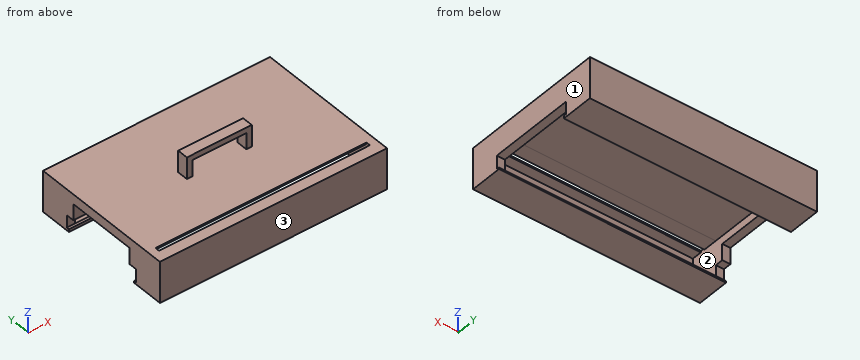
Solid Edge part; units mm, degrees
sketch "Sketch1" plane through (0, 0, 0) normal (0, 0, 1) x (1, 0, 0)
  line L0 (-210, -135) -> (210, -135)
  line L1 (210, -135) -> (210, 135)
  line L2 (210, 135) -> (-210, 135)
  line L3 (-210, 135) -> (-210, -135)
extrude "Protrusion1" add sketch "Sketch1" along normal blind 76
sketch "Sketch2" plane through (0, 0, 0) normal (0, 0, -1) x (1, 0, 0)
  line L0 (-195, 80) -> (195, 80)
  line L1 (195, 80) -> (195, -80)
  line L2 (195, -80) -> (-195, -80)
  line L3 (-195, -80) -> (-195, 80)
extrude "ExtrudedCutout_1" cut sketch "Sketch2" against normal blind 70
sketch "Sketch3" plane through (0, -80, 35) normal (0, 1, 0) x (-1, 0, 0)
  line L0 (195, -32) -> (-195, -32)
  line L1 (-195, -32) -> (-195, 38)
  line L2 (-195, 38) -> (195, 38)
  line L3 (195, 38) -> (195, -32)
extrude "ExtrudedCutout_2" cut sketch "Sketch3" against normal blind 53
sketch "Sketch4" plane through (210, 0, 38) normal (1, 0, 0) x (0, 1, 0)
  line L0 (80, -10) -> (-80, -10)
  line L1 (-80, -10) -> (-80, -38)
  line L2 (-80, -38) -> (80, -38)
  line L3 (80, -38) -> (80, -10)
extrude "Cutout1" cut sketch "Sketch4" against normal through all
sketch "Sketch5" plane through (0, 0, 70) normal (0, 0, -1) x (0, 1, 0)
  line L0 (80, -195) -> (-80, -195)
  line L1 (-80, -195) -> (-80, 195)
  line L2 (-80, 195) -> (80, 195)
  line L3 (80, 195) -> (80, -195)
extrude "ExtrudedCutout_5" cut sketch "Sketch5" against normal blind 2.5929
sketch "Sketch6" plane through (0, 0, 70) normal (0, 0, -1) x (0, 1, 0)
  line L0 (80, -195) -> (-80, -195)
  line L1 (-80, -195) -> (-80, 195)
  line L2 (-80, 195) -> (80, 195)
  line L3 (80, 195) -> (80, -195)
extrude "ExtrudedCutout_6" cut sketch "Sketch6" against normal blind 2.9454
sketch "Sketch7" plane through (0, 0, 76) normal (0, 0, 1) x (1, 0, 0)
  line L0 (-60, -10) -> (60, -10)
  line L1 (60, -10) -> (60, 10)
  line L2 (60, 10) -> (-60, 10)
  line L3 (-60, 10) -> (-60, -10)
extrude "ExtrudedProtrusion_2" add sketch "Sketch7" along normal blind 40
sketch "Sketch8" plane through (0, -10, 96) normal (0, -1, 0) x (1, 0, 0)
  line L0 (-50, 10) -> (50, 10)
  line L1 (50, 10) -> (50, -20)
  line L2 (50, -20) -> (-50, -20)
  line L3 (-50, -20) -> (-50, 10)
extrude "Cutout2" cut sketch "Sketch8" against normal up to next
sketch "Sketch9" plane through (0, 0, 76) normal (0, 0, 1) x (1, 0, 0)
  line L0 (195, -114.1043) -> (-195, -114.1043)
  line L1 (-195, -114.1043) -> (-195, -106.1043)
  line L2 (-195, -106.1043) -> (195, -106.1043)
  line L3 (195, -106.1043) -> (195, -114.1043)
extrude "Cutout3" cut sketch "Sketch9" against normal up to next
sketch "Sketch10" plane through (210, 0, 38) normal (1, 0, 0) x (0, 1, 0)
  line L0 (-75, -38) -> (-75, -35)
  line L1 (-75, -35) -> (-80, -35)
  line L2 (-80, -35) -> (-80, -38)
  line L3 (-80, -38) -> (-75, -38)
  line L4 (75, -38) -> (75, -33)
  line L5 (75, -33) -> (80, -33)
  line L6 (80, -33) -> (80, -38)
  line L7 (80, -38) -> (75, -38)
extrude "ExtrudedProtrusion_3" add sketch "Sketch10" against normal blind 420
sketch "Sketch11" plane through (0, 80, 38.9727) normal (0, -1, 0) x (1, 0, 0)
  line L0 (195, 34.0273) -> (195, -35.9727)
  line L1 (195, -35.9727) -> (-195, -35.9727)
  line L2 (-195, -35.9727) -> (-195, 34.0273)
  line L3 (-195, 34.0273) -> (195, 34.0273)
extrude "Cutout4" cut sketch "Sketch11" against normal blind 50.6298
sketch "Sketch12" plane through (-210, 0, 38) normal (-1, 0, 0) x (0, -1, 0)
  line L0 (65, 20) -> (-65, 20)
  line L1 (-65, 20) -> (-65, -10)
  line L2 (-65, -10) -> (65, -10)
  line L3 (65, -10) -> (65, 20)
extrude "Cutout5" cut sketch "Sketch12" against normal up to next
sketch "Sketch13" plane through (-195, -1.1851, 39.5) normal (1, 0, 0) x (0, 1, 0)
  line L0 (66.1851, 36.5) -> (66.1851, -11.5)
  line L1 (66.1851, -11.5) -> (81.1851, -11.5)
  line L2 (81.1851, -11.5) -> (81.1851, 36.5)
  line L3 (81.1851, 36.5) -> (66.1851, 36.5)
extrude "Protrusion2" add sketch "Sketch13" along normal blind 400.6236
properties material "Polycarbonate"
Design review of the part built by this model. Coordinates are the model's own, in mm. Face numbers are marked on the shaded views. Coordinates: 2 decimals unless noted, no trailing zeros. Write each loop counter-clockwise with the first axis right and the second up, starting at its lowest first coordinate (ties: lowest second). Pieces come first, ordered by that corner, then holes. Notation, with made-up numbers: (-12, 10.5) - (45, 10.5) arc R10 ccw to (45, 16.5) - close; hole circle Ø1 at (17, 57.25). An arc over 180 degrees is marked (long way). Use one line per item in the form item = value.
Q1. The part is to be moulded in two halves that separate along X. For the marked faces 1, 2 and 3, say which applies: +X half, -X half, draft (parallel to the pull), parting line (faces both ways), or undercut.
Taken from the geometry:
face_1 = +X half
face_2 = undercut
face_3 = draft
Q2. Insertion check: pin 1 Ø6 at (y, z) = (-11, 23.5) entering from +X; pin 2 Ø4.5 at (x, y) = (-200.5, -17.5) entering from -Z; pin 3 Ø4 at (x, y) = (-151, 91) entering from +Z; pin 4 Ø22 at (y, z) = (-4, 92.5) entering from -X. Each pin has a flat end and moves straight along its axis. Give the tip position at first contact, or say it passes through.
Taken from the geometry:
pin_1 = through
pin_2 = 58
pin_3 = 76
pin_4 = -60
Q3. Consider section A-A (z = 45.5). Write out the cut boundary in (x, y), plus the area to 3 significant figures.
Taken from the geometry:
outline = (-210, -135) - (210, -135) - (210, 135) - (-210, 135) - (-210, 65) - (195, 65) - (195, -133) - (-195, -133) - (-195, -65) - (-210, -65) - close; hole (-195, 80) - (195, 80) - (195, 130.63) - (-195, 130.63) - close
area = 14,500 mm^2
Q4. For probe 1 along Y at (x, z) = (-144, 66); probe 2 along X at (y, z) = (-82.5, 54); probe 3 along X at (y, z) = (8.5, 103), list the stretches that pass through material, from the lowest coordinate up.
Taken from the geometry:
probe_1 = -135 to -133, 65 to 80, 130.63 to 135
probe_2 = -210 to -195, 195 to 210
probe_3 = -60 to -50, 50 to 60
Q5. Consider section D-D (y = 103.5). Write out the cut boundary in (x, z).
Taken from the geometry:
outline = (-210, 0) - (210, 0) - (210, 76) - (-210, 76) - close; hole (-195, 3) - (195, 3) - (195, 73) - (-195, 73) - close
Q6. Consider section C-C (z = 11.5). Write out the cut boundary in (x, y), plus the area to 3 significant figures.
Taken from the geometry:
outline = (-210, -135) - (210, -135) - (210, -80) - (195, -80) - (195, -133) - (-195, -133) - (-195, -80) - (-210, -80) - close; (-210, 80) - (-195, 80) - (-195, 130.63) - (195, 130.63) - (195, 80) - (210, 80) - (210, 135) - (-210, 135) - close
area = 5,780 mm^2
Q7. Consider section B-B (x = -69). Write out the cut boundary in (y, z), plus the area to 3 significant figures.
Taken from the geometry:
outline = (-135, 0) - (-75, 0) - (-75, 3) - (-133, 3) - (-133, 73) - (-114.1, 73) - (-114.1, 76) - (-135, 76) - close; (-106.1, 73) - (-80, 73) - (-80, 72.95) - (65, 72.95) - (65, 28) - (80, 28) - (80, 73) - (130.63, 73) - (130.63, 3) - (80, 3) - (80, 5) - (75, 5) - (75, 0) - (135, 0) - (135, 76) - (-106.1, 76) - close
area = 2,280 mm^2
